Part model, mm, in its own coordinate system. A direction names the side the tool comes from. Round coordinates to 2 decimals unless told otherwise and drop trailing zeros. Order: outer loops, then holes, each group sorted by start corner. A loop starts at its lowest first (then second) coordinate and runs counter-clockwise, first axis right, second up. Notation, with made-up numbers: (67, 1.5) - (85, 1.5) arc R12 ccw to (85, 5.5) - close; hole circle Ø7 at (-27, -28.5). An arc over 180 degrees is marked (long way). Return JSON: item names as keys, results as strings. Group by question number.
Item 1: Probe probe 1 along Y at (x, z) = (-105, 3.5); probe 2 along X at (y, z) = (-172.5, 7.5); probe 3 along X at (y, z) = (175, 4). List the from-to ranges inside material, lowest first.
Item 2: Tool access for faces 1 (the face through (185, -2, 5)), 2 (the face through (135, 2, 5)): list every direction of +Z, -Z, +X, -X, +Y, -Y with a clear straight run to the whole face (end or side of a thin tool).
Item 3: Saw through at C-C on z = 1.75. State how many separate pieces and enclosed holes the cut face has, and give its area (3 significant figures).
Item 4: Two-plate mould, pull along Y, no slides. Class faces 3 (the face through (180, 180, 5)), 4 (the face through (180, -180, 5)), 5 (the face through (-44, -135, 5)): released by +Y, released by -Y, zero draft, split by the parting line, or undercut.
Item 5: Saw through at A-A on x = -114. List the corners of the cut face in (y, z), and give its area (3 significant figures).
```python
from build123d import *

# Parameters (mm, degrees)
SKETCH1_W           = 370
SKETCH1_H           = 370
SKETCH1_R           = 3.2
SKETCH1_R_2         = 1.5
BOSS_EXTRUDE1_DEPTH = 10
CHAMFER1_SIZE       = 10
CUT_EXTRUDE1_DEPTH  = 10


with BuildPart() as part:
    # Sketch1 → Boss-Extrude1 (new body)
    with BuildSketch(Plane.XY):
        Rectangle(SKETCH1_W, SKETCH1_H)
        with Locations((85, -152.5)):
            Circle(SKETCH1_R, mode=Mode.SUBTRACT)
        with Locations((85, -172.5)):
            Circle(SKETCH1_R, mode=Mode.SUBTRACT)
        with Locations((105, -152.5)):
            Circle(SKETCH1_R, mode=Mode.SUBTRACT)
        with Locations((105, -172.5)):
            Circle(SKETCH1_R, mode=Mode.SUBTRACT)
        with Locations((-105, -172.5)):
            Circle(SKETCH1_R, mode=Mode.SUBTRACT)
        with Locations((-105, -152.5)):
            Circle(SKETCH1_R, mode=Mode.SUBTRACT)
        with Locations((-85, -172.5)):
            Circle(SKETCH1_R, mode=Mode.SUBTRACT)
        with Locations((-85, -152.5)):
            Circle(SKETCH1_R, mode=Mode.SUBTRACT)
        with Locations((155, -145)):
            Circle(SKETCH1_R_2, mode=Mode.SUBTRACT)
        with Locations((175, -145)):
            Circle(SKETCH1_R_2, mode=Mode.SUBTRACT)
        with Locations((165, -165)):
            Circle(SKETCH1_R_2, mode=Mode.SUBTRACT)
        with Locations((-155, -145)):
            Circle(SKETCH1_R_2, mode=Mode.SUBTRACT)
        with Locations((-175, -145)):
            Circle(SKETCH1_R_2, mode=Mode.SUBTRACT)
        with Locations((-165, -165)):
            Circle(SKETCH1_R_2, mode=Mode.SUBTRACT)
        with Locations((155, 175)):
            Circle(SKETCH1_R_2, mode=Mode.SUBTRACT)
        with Locations((175, 175)):
            Circle(SKETCH1_R_2, mode=Mode.SUBTRACT)
        with Locations((-155, 175)):
            Circle(SKETCH1_R_2, mode=Mode.SUBTRACT)
        with Locations((-175, 175)):
            Circle(SKETCH1_R_2, mode=Mode.SUBTRACT)
        Polygon((-135, 135), (135, 135), (135, -135), (20, -135), (10, -155), (-10, -155), (-20, -135), (-135, -135), align=None, mode=Mode.SUBTRACT)
    extrude(amount=BOSS_EXTRUDE1_DEPTH)

    # Chamfer1
    chamfer1_edges = [part.edges().sort_by_distance(p)[0] for p in [
        (135, -135, 5),
        (135, 135, 5),
        (-135, 135, 5),
        (-135, -135, 5),
        (-185, -185, 5),
        (-185, 185, 5),
        (185, 185, 5),
        (185, -185, 5),
    ]]
    chamfer(chamfer1_edges, length=CHAMFER1_SIZE)

    # Sketch2 → Cut-Extrude1 (cut)
    with BuildSketch(Plane.XY.offset(10)):
        Polygon((-101, -135), (-95, -141), (-75, -141), (-69, -135), align=None)
        Polygon((75, -141), (69, -135), (101, -135), (95, -141), align=None)
    extrude(amount=-CUT_EXTRUDE1_DEPTH, mode=Mode.SUBTRACT)


solid = part.part
```
Filled in:
{
 "1": {"probe 1": "y = -185 to -175.7, -169.3 to -155.7, -149.3 to -135, 135 to 185", "probe 2": "x = -185 to -108.2, -101.8 to -88.2, -81.8 to 81.8, 88.2 to 101.8, 108.2 to 185", "probe 3": "x = -185 to -176.5, -173.5 to -156.5, -153.5 to 153.5, 156.5 to 173.5, 176.5 to 185"},
 "2": {"face 1": "+Z, -Z, +X, +Y, -Y", "face 2": "+Z, -Z"},
 "3": {"separate pieces": "1", "enclosed holes": "19", "area": "62,800 mm^2"},
 "4": {"face 3": "released by +Y", "face 4": "released by -Y", "face 5": "undercut"},
 "5": {"outline": "(-185, 0) - (-135, 0) - (-135, 10) - (-185, 10) - close; (135, 0) - (185, 0) - (185, 10) - (135, 10) - close", "area": "1,000 mm^2"}
}
